Input: part model. Units: mm. Frame: model coordinates. A direction names the side the tool comes from. Give positions to 0.01 mm unless a question says otherwise; leave off trailing zeros. Loops run counter-clockwise (first coordinate to the right, second up) from the corner with the lowest first, then second, coordinate; pieces in that order, holes last. Notation, with made-up numbers: (-32.75, 18.5) -> (14.25, 18.5) arc R19 ccw to (14.25, 37.5) -> close; hole circle Ø6 at (-33, -15.75). An arc over 180 degrees is marked (long way). One line per question, with ' | ' between items.
from build123d import *

# Parameters (mm, degrees)
SKETCH1_W           = 86.36
SKETCH1_H           = 31.75
BOSS_EXTRUDE1_DEPTH = 16.764
SKETCH2_W           = 25.4
SKETCH2_H           = 6.35
CUT_EXTRUDE1_DEPTH  = 86.36
SKETCH3_W           = 25.4
SKETCH3_H           = 6.35
CUT_EXTRUDE2_DEPTH  = 50.8
SKETCH5_W           = 61.722
SKETCH5_H           = 17.1196
CUT_EXTRUDE3_DEPTH  = 1.016
SKETCH5_3_R         = 0.81915
CUT_EXTRUDE4_DEPTH  = 49.964882528
CUT_EXTRUDE8_REACH  = 58.157
SKETCH6_W           = 10.16
SKETCH6_H           = 5.08
SKETCH6_R           = 0.8255
SKETCH6_H_2         = 6.985
SKETCH6_H_3         = 2.1717
SKETCH7_W           = 25.4
SKETCH7_H           = 7.62
BOSS_EXTRUDE2_DEPTH = 25.4
CUT_EXTRUDE9_DEPTH  = 25.4
FILLET1_R           = 0.381
SKETCH11_W          = 25.4
SKETCH11_H          = 8.89
BOSS_EXTRUDE5_DEPTH = 31.75
FILLET2_R           = 0.762
CUT_EXTRUDE10_DEPTH = 25.4
FILLET4_R           = 5.08
SKETCH10_R          = 2.7051
CUT_EXTRUDE11_DEPTH = 8.001


with BuildPart() as part:
    # Sketch1 → Boss-Extrude1 (new body)
    with BuildSketch(Plane(origin=(0, 0, 0), x_dir=(1, 0, 0), z_dir=(0, 1, 0))):
        Rectangle(SKETCH1_W, SKETCH1_H)
    extrude(amount=BOSS_EXTRUDE1_DEPTH)

    # Sketch2 → Cut-Extrude1 (cut)
    with BuildSketch(Plane.ZY.offset(43.18)):
        with Locations((-3.175, 7.239)):
            Rectangle(SKETCH2_W, SKETCH2_H)
    extrude(amount=-CUT_EXTRUDE1_DEPTH, mode=Mode.SUBTRACT)

    # Sketch3 → Cut-Extrude2 (cut)
    with BuildSketch(Plane.ZY.offset(43.18)):
        with Locations((-3.175, 13.589)):
            Rectangle(SKETCH3_W, SKETCH3_H)
    cut_extrude2 = extrude(amount=-CUT_EXTRUDE2_DEPTH, mode=Mode.SUBTRACT)

    # Mirror1: Cut-Extrude2 across plane
    add(cut_extrude2.mirror(Plane(origin=(0, 0, 0), x_dir=(0, 0, 1), z_dir=(1, 0, 0))), mode=Mode.SUBTRACT)

    # Sketch5 → Cut-Extrude3 (cut)
    with BuildSketch(Plane.XZ):
        with Locations((0, 7.3152)):
            Rectangle(SKETCH5_W, SKETCH5_H)
    extrude(amount=-CUT_EXTRUDE3_DEPTH, mode=Mode.SUBTRACT)

    # Sketch5<3> → Cut-Extrude4 (cut, through all)
    with BuildSketch(Plane.XZ):
        with Locations(Location((-27.9908, 1.2954, 0), (0, 0, 270))):
            Circle(SKETCH5_3_R)
        with Locations(Location((27.9908, 1.2954, 0), (0, 0, 270))):
            Circle(SKETCH5_3_R)
    extrude(amount=-CUT_EXTRUDE4_DEPTH, mode=Mode.SUBTRACT)

    # Cut-Extrude8: up to this face of the body (flat: up to its plane)
    cut_extrude8_end = Plane(part.part.faces().sort_by_distance((0, 2.032, -15.875))[0])
    # Sketch6 → Cut-Extrude8 (cut, up to the picked face)
    with BuildSketch(Plane.XY.offset(15.875), mode=Mode.PRIVATE) as cut_extrude8_sk1:
        with Locations((38.1, 12.0523)):
            Rectangle(SKETCH6_W, SKETCH6_H)
        with Locations((40.9448, 12.6873)):
            Circle(SKETCH6_R, mode=Mode.SUBTRACT)
    cut_extrude8_tool1 = split(extrude(cut_extrude8_sk1.sketch, amount=-CUT_EXTRUDE8_REACH, mode=Mode.PRIVATE), bisect_by=cut_extrude8_end, keep=Keep.BOTH, mode=Mode.PRIVATE)
    # Sketch6 → Cut-Extrude8 (cut, up to the picked face)
    with BuildSketch(Plane.XY.offset(15.875), mode=Mode.PRIVATE) as cut_extrude8_sk2:
        with Locations((40.9448, 12.6873)):
            Circle(SKETCH6_R)
    cut_extrude8_tool2 = split(extrude(cut_extrude8_sk2.sketch, amount=-CUT_EXTRUDE8_REACH, mode=Mode.PRIVATE), bisect_by=cut_extrude8_end, keep=Keep.BOTH, mode=Mode.PRIVATE)
    # Sketch6 → Cut-Extrude8 (cut, up to the picked face)
    with BuildSketch(Plane.XY.offset(15.875), mode=Mode.PRIVATE) as cut_extrude8_sk3:
        with Locations((17.3355, 12.6873)):
            Circle(SKETCH6_R)
    cut_extrude8_tool3 = split(extrude(cut_extrude8_sk3.sketch, amount=-CUT_EXTRUDE8_REACH, mode=Mode.PRIVATE), bisect_by=cut_extrude8_end, keep=Keep.BOTH, mode=Mode.PRIVATE)
    # Sketch6 → Cut-Extrude8 (cut, up to the picked face)
    with BuildSketch(Plane.XY.offset(15.875), mode=Mode.PRIVATE) as cut_extrude8_sk4:
        with Locations((40.9448, 5.715)):
            Circle(SKETCH6_R)
    cut_extrude8_tool4 = split(extrude(cut_extrude8_sk4.sketch, amount=-CUT_EXTRUDE8_REACH, mode=Mode.PRIVATE), bisect_by=cut_extrude8_end, keep=Keep.BOTH, mode=Mode.PRIVATE)
    # Sketch6 → Cut-Extrude8 (cut, up to the picked face)
    with BuildSketch(Plane.XY.offset(15.875), mode=Mode.PRIVATE) as cut_extrude8_sk5:
        with Locations((-38.1, 3.4925)):
            Rectangle(SKETCH6_W, SKETCH6_H_2)
        with Locations((-40.9448, 5.715)):
            Circle(SKETCH6_R, mode=Mode.SUBTRACT)
    cut_extrude8_tool5 = split(extrude(cut_extrude8_sk5.sketch, amount=-CUT_EXTRUDE8_REACH, mode=Mode.PRIVATE), bisect_by=cut_extrude8_end, keep=Keep.BOTH, mode=Mode.PRIVATE)
    # Sketch6 → Cut-Extrude8 (cut, up to the picked face)
    with BuildSketch(Plane.XY.offset(15.875), mode=Mode.PRIVATE) as cut_extrude8_sk6:
        with Locations((-40.9448, 5.715)):
            Circle(SKETCH6_R)
    cut_extrude8_tool6 = split(extrude(cut_extrude8_sk6.sketch, amount=-CUT_EXTRUDE8_REACH, mode=Mode.PRIVATE), bisect_by=cut_extrude8_end, keep=Keep.BOTH, mode=Mode.PRIVATE)
    # Sketch6 → Cut-Extrude8 (cut, up to the picked face)
    with BuildSketch(Plane.XY.offset(15.875), mode=Mode.PRIVATE) as cut_extrude8_sk7:
        with Locations((-17.3355, 5.715)):
            Circle(SKETCH6_R)
    cut_extrude8_tool7 = split(extrude(cut_extrude8_sk7.sketch, amount=-CUT_EXTRUDE8_REACH, mode=Mode.PRIVATE), bisect_by=cut_extrude8_end, keep=Keep.BOTH, mode=Mode.PRIVATE)
    # Sketch6 → Cut-Extrude8 (cut, up to the picked face)
    with BuildSketch(Plane.XY.offset(15.875), mode=Mode.PRIVATE) as cut_extrude8_sk8:
        with Locations((-40.9448, 12.6873)):
            Circle(SKETCH6_R)
    cut_extrude8_tool8 = split(extrude(cut_extrude8_sk8.sketch, amount=-CUT_EXTRUDE8_REACH, mode=Mode.PRIVATE), bisect_by=cut_extrude8_end, keep=Keep.BOTH, mode=Mode.PRIVATE)
    # Sketch6 → Cut-Extrude8 (cut, up to the picked face)
    with BuildSketch(Plane.XY.offset(15.875), mode=Mode.PRIVATE) as cut_extrude8_sk9:
        with Locations((38.1, 15.67815)):
            Rectangle(SKETCH6_W, SKETCH6_H_3)
    cut_extrude8_tool9 = split(extrude(cut_extrude8_sk9.sketch, amount=-CUT_EXTRUDE8_REACH, mode=Mode.PRIVATE), bisect_by=cut_extrude8_end, keep=Keep.BOTH, mode=Mode.PRIVATE)
    add(cut_extrude8_tool1.solids().sort_by(Axis((37.976895, 12.024821, 15.875), (0, 0, -1)))[0], mode=Mode.SUBTRACT)
    add(cut_extrude8_tool2.solids().sort_by(Axis((40.9448, 12.6873, 15.875), (0, 0, -1)))[0], mode=Mode.SUBTRACT)
    add(cut_extrude8_tool3.solids().sort_by(Axis((17.3355, 12.6873, 15.875), (0, 0, -1)))[0], mode=Mode.SUBTRACT)
    add(cut_extrude8_tool4.solids().sort_by(Axis((40.9448, 5.715, 15.875), (0, 0, -1)))[0], mode=Mode.SUBTRACT)
    add(cut_extrude8_tool5.solids().sort_by(Axis((-38.011513, 3.42337, 15.875), (0, 0, -1)))[0], mode=Mode.SUBTRACT)
    add(cut_extrude8_tool6.solids().sort_by(Axis((-40.9448, 5.715, 15.875), (0, 0, -1)))[0], mode=Mode.SUBTRACT)
    add(cut_extrude8_tool7.solids().sort_by(Axis((-17.3355, 5.715, 15.875), (0, 0, -1)))[0], mode=Mode.SUBTRACT)
    add(cut_extrude8_tool8.solids().sort_by(Axis((-40.9448, 12.6873, 15.875), (0, 0, -1)))[0], mode=Mode.SUBTRACT)
    add(cut_extrude8_tool9.solids().sort_by(Axis((38.1, 15.67815, 15.875), (0, 0, -1)))[0], mode=Mode.SUBTRACT)

    # Sketch7 → Boss-Extrude2 (add)
    with BuildSketch(Plane(origin=(0, 0, 9.525), x_dir=(-1, 0, 0), z_dir=(0, 0, -1))):
        with Locations((0, 12.954)):
            Rectangle(SKETCH7_W, SKETCH7_H)
    extrude(amount=BOSS_EXTRUDE2_DEPTH)

    # Sketch8 → Cut-Extrude9 (cut)
    with BuildSketch(Plane.ZY.offset(12.7)):
        Polygon((-15.875, 10.287), (9.525, 10.668), (9.525, 9.144), (-15.875, 9.144), align=None)
    extrude(amount=-CUT_EXTRUDE9_DEPTH, mode=Mode.SUBTRACT)

    # Fillet1
    fillet1_edges = [part.edges().sort_by_distance(p)[0] for p in [
        (0, 10.668, 9.525),
    ]]
    fillet(fillet1_edges, radius=FILLET1_R)

    # Sketch11 → Boss-Extrude5 (add)
    with BuildSketch(Plane.XY.offset(15.875)):
        with Locations((0, 21.209)):
            Rectangle(SKETCH11_W, SKETCH11_H)
    extrude(amount=-BOSS_EXTRUDE5_DEPTH)

    # Fillet2
    fillet2_edges = [part.edges().sort_by_distance(p)[0] for p in [
        (-31.9405, 0, 15.875),
        (-38.1, 6.985, 15.875),
        (38.1, 9.5123, 15.875),
        (-27.94, 16.764, 15.875),
        (22.86, 16.764, 15.875),
        (5.08, 0, -15.875),
        (37.0205, 0, 15.875),
    ]]
    fillet(fillet2_edges, radius=FILLET2_R)

    # Sketch12 → Cut-Extrude10 (cut)
    with BuildSketch(Plane.ZY.offset(12.7)):
        with BuildLine():
            Line((-15.875, 16.764), (-15.875, 25.654))
            Line((-15.875, 25.654), (15.875, 25.654))
            Line((15.875, 25.654), (15.875, 24.911939438))
            ThreePointArc((15.875, 24.911939438), (9.270292434, 25.222373256), (2.900847527, 23.447914815))
            ThreePointArc((2.900847527, 23.447914815), (-6.338198623, 19.687743912), (-15.875, 16.764))
        make_face()
    extrude(amount=-CUT_EXTRUDE10_DEPTH, mode=Mode.SUBTRACT)

    # Fillet4
    fillet4_edges = [part.edges().sort_by_distance(p)[0] for p in [
        (-12.7, 19.687743912, -6.338198623),
        (-12.7, 25.222373256, 9.270292434),
        (12.7, 19.687743912, -6.338198623),
        (12.7, 25.222373256, 9.270292434),
    ]]
    fillet(fillet4_edges, radius=FILLET4_R)

    # Sketch10 → Cut-Extrude11 (cut)
    with BuildSketch(Plane.XY.offset(15.875)):
        with Locations((0, 20.828)):
            Circle(SKETCH10_R)
    extrude(amount=-CUT_EXTRUDE11_DEPTH, mode=Mode.SUBTRACT)


solid = part.part
1. Pin query (flat end, axial travel): P1, Ø6, axis at x = -24, z = 12, coming from the +Y side; P2, Ø10, axis at y = 3, z = -12, coming from the -X side; P3, Ø11, axis at y = 15, z = 3.5, coming from the -X side; P4, Ø6, axis at y = 5, z = 9, coming from the -X side. Return the tip coordinate at first contact, or that it passes through.
Determined:
P1: stops at y = 16.76 | P2: stops at x = -33.02 | P3: stops at x = -12.7 | P4: stops at x = -43.18
2. Ray query, line 1 along X through (y, z) = (11, -10.5); line 2 along Y through (x, z) = (-27, 0); line 3 along Y through (x, z) = (-5.5, 2.5). Return the intervals inside material, ascending. Write a range as from..to.
Determined:
line 1: x = -12.7..12.7 | line 2: y = 1.02..4.06 | line 3: y = 1.02..4.06, 10.56..23.26
3. Pull-direction query (Z, two-part tool) for faces 1 (the cylindrical face through (27.19, 2.52, 1.47)), 2 (the cylindrical face through (-0.107, 25.233, 9.363)), 3 (the flat face through (-33.02, 2, 0)), 4 (the cylindrical face through (-27.18, 2.52, 1.4)); classes: pulls with the +Z half, pulls with the -Z half, needs draft (parallel to the pull), parting line crosses it, or undercut.
Determined:
face 1: undercut | face 2: parting line crosses it | face 3: needs draft | face 4: undercut
4. Section query B-B (z = 14). Count the separate pieces of the cut face and the enclosed holes in it, then the cut area to 3 significant figures.
Determined:
separate pieces: 1 | enclosed holes: 5 | area: 1,410 mm2
5. Section query A-A (x = 0). Output: boundary loops of the cut face in (y, z) (3 decimals).
Determined:
outline: (0, -15.113) arc R0.762 ccw to (0.762, -15.875) -> (4.064, -15.875) -> (4.064, 9.525) -> (10.281, 9.525) arc R0.381 cw to (10.662, 9.138) -> (10.287, -15.875) -> (16.764, -15.875) arc R112.068 cw to (23.448, 2.901) arc R20.837 ccw to (24.912, 15.875) -> (23.533, 15.875) -> (23.533, 7.874) -> (18.123, 7.874) -> (18.123, 15.875) -> (1.016, 15.875) -> (1.016, -1.245) -> (0, -1.245) -> close
6. Section query C-C (x = -34.5). Output: boundary loops of the cut face in (y, z) (3 decimals), then the cut area to 3 significant figures.
Determined:
outline: (6.985, 9.525) -> (16.764, 9.525) -> (16.764, 15.113) arc R0.762 ccw to (16.002, 15.875) -> (7.747, 15.875) arc R0.762 ccw to (6.985, 15.113) -> close | area: 61.8 mm2
7. Reachability of faces 5 (the flat face through (0, 21, 7.874)), 6 (the flat face through (23, 16.764, 12)), 7 (the flat face through (-28, 16.764, 12)), 8 (the flat face through (0, 1.016, 7)) from +Z, -Z, +X, -X, +Y, -Y: full face, straight path, thin tool, end or side. Return the list, or none.
Determined:
face 5: +Z | face 6: +Z, -Z, +X, +Y | face 7: +Z, -Z, -X, +Y | face 8: +Z, -Y
8. Section query D-D (x = 10). Output: boundary loops of the cut face in (y, z) (3 decimals).
Determined:
outline: (0, -15.113) arc R0.762 ccw to (0.762, -15.875) -> (4.064, -15.875) -> (4.064, 9.525) -> (10.281, 9.525) arc R0.381 cw to (10.662, 9.138) -> (10.287, -15.875) -> (16.153, -15.875) arc R112.66 cw to (22.91, 3.148) arc R20.245 ccw to (24.307, 15.875) -> (1.016, 15.875) -> (1.016, -1.245) -> (0, -1.245) -> close
